Design review of the part built by this model. Coordinates are the model's own, in mm. Face numbers are marked on the shaded views. A direction names the side the tool comes from. Coordinates: 2 decimals unless noted, no trailing zeros. Loops run counter-clockwise (first coordinate to the right, second up) from the corner with the lowest first, then second, coordinate; pieces in that order, holes last. Notation, with made-up numbers: M -7.5,-26 L 3.5,-26 A14 cw 3.5,-5 Z; hole C 83,2 d3. An arc over 180 degrees is marked long. Put each result on its own line as item: value. Start each with the question number.
(1) Clearance check with flat-ended pins moving along their axes: pin 1 (2 mm diameter, centred on x = 2.5, z = 1.5, fed in from -Y); pin 2 (3.5 mm diameter, centred on x = -3.94, y = 8.65, fed in from +Z); pin 3 (0.9 mm diameter, centred on x = 1, z = 1, fed in from +Y); pin 4 (3 mm diameter, centred on y = 11.5, z = 1, fed in from +X). State where each tip first meets the part, or that it passes through.
(2) For the marked faces 5, 6, 7 and 8, list the 3-axis set-ups (+Z, -Z, +X, -X, +Y, -Y) from which the entire face can be reached by the end or side of a thin tool; tool diameter is ignored.
(3) Take a section at C-C, the plane y = 7.5. Give the boundary of the cut face in (x, z).
(4) Take a section at A-A, the plane x = -3.5. Give the boundary of the cut face in (y, z), then the cut area to 3 significant figures.
(5) The part is to be moulded in two halves that separate along Y. For the marked faces 1, 2, 3 and 4, say which applies: +Y half, -Y half, draft (parallel to the pull), parting line (faces both ways), or undercut.
(6) Take a section at D-D, the plane z = 1. Give the boundary of the cut face in (x, y), then the cut area to 3 significant figures.
(7) For probe 1 along X at (y, z) = (9.5, 0.25); probe 2 along X at (y, z) = (8, -1); probe 3 along Y at (x, z) = (-3.75, -3), list the stretches that pass through material, from the lowest coordinate up. Write a range as [from, to].
(8) Take a section at B-B, the plane z = -0.75. Give the boundary of the cut face in (x, y).
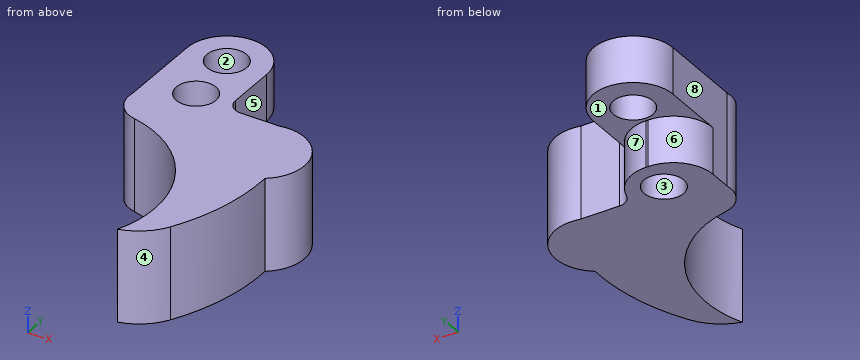
```python
from build123d import *

# Parameters (mm, degrees)
BOSS_EXTRUDE1_DEPTH      = 3.5
BOSS_EXTRUDE1_DEPTH_BACK = 3.5
SKETCH6_R                = 1.5
CUT_EXTRUDE1_DEPTH       = 19.96660999
SKETCH7_W                = 4.034122634
SKETCH7_H                = 6.882168449
CUT_EXTRUDE2_DEPTH       = 18.97170817
FILLET1_R                = 3
CUT_EXTRUDE3_DEPTH       = 18.97170817
CUT_EXTRUDE3_DEPTH_BACK  = 18.97170817
SKETCH5_R                = 1.5


with BuildPart() as part:
    # Sketch1 → Boss-Extrude1 (new, two sides: drawn at the far end of the back side and taken through both)
    with BuildSketch(Plane.XY.offset(-BOSS_EXTRUDE1_DEPTH_BACK)):
        with BuildLine():
            Line((-7.379331989, 6.554089817), (-7.379331989, 12.992324067))
            ThreePointArc((-7.379331989, 12.992324067), (-4.379331989, 15.992324067), (-1.379331989, 12.992324067))
            Line((-1.379331989, 12.992324067), (-1.379331989, 9.288226288))
            ThreePointArc((-1.379331989, 9.288226288), (-1.067058002, 8.534330194), (-0.313161909, 8.222056208))
            Line((-0.313161909, 8.222056208), (2.596292865, 8.222056208))
            ThreePointArc((2.596292865, 8.222056208), (6.230009224, 6.392230094), (5.19642183, 2.457277072))
            ThreePointArc((5.19642183, 2.457277072), (4.763363262, -1.740328915), (3.218784408, -5.667377669))
            ThreePointArc((3.218784408, -5.667377669), (2.087900651, -6.964096239), (0.531658525, -7.697913361))
            ThreePointArc((0.531658525, -7.697913361), (0.209560398, -0.37433078), (-5.652587934, 4.027240071))
            ThreePointArc((-5.652587934, 4.027240071), (-7.035324124, 4.93575307), (-7.379331989, 6.554089817))
        make_face()
    extrude(amount=BOSS_EXTRUDE1_DEPTH + BOSS_EXTRUDE1_DEPTH_BACK)

    # Sketch6 → Cut-Extrude1 (cut, through all)
    with BuildSketch(Plane.XY.offset(3.5)):
        with Locations((-4.379331989, 12.992324067)):
            Circle(SKETCH6_R)
    extrude(amount=-CUT_EXTRUDE1_DEPTH, mode=Mode.SUBTRACT)

    # Sketch7 → Cut-Extrude2 (cut, through all)
    with BuildSketch(Plane(origin=(0, 0, 0), x_dir=(0, 0, -1), z_dir=(1, 0, 0))):
        with Locations((2.017061317, 14.662562736)):
            Rectangle(SKETCH7_W, SKETCH7_H)
    extrude(amount=-CUT_EXTRUDE2_DEPTH, mode=Mode.SUBTRACT)

    # Fillet1
    # the kernel refuses this fillet: 3 mm, written as the material it takes off along each edge
    with BuildSketch(Plane(origin=(-7.379331989, 11.221478511, 0), x_dir=(0, -1, 0), z_dir=(0, 0, -1))) as fillet1_piece_1:
        with BuildLine():
            CenterArc((FILLET1_R, -FILLET1_R), FILLET1_R, 90, 90)
            Line((0, -FILLET1_R), (0, 0))
            Line((0, 0), (FILLET1_R, 0))
        make_face()
    extrude(amount=11, mode=Mode.SUBTRACT)
    with BuildSketch(Plane(origin=(-1.379331989, 11.221478511, -10.643941593), x_dir=(0.016872794888794368, -0.9998576442637425, 0), z_dir=(0, 0, 1))) as fillet1_piece_2:
        with BuildLine():
            CenterArc((2.951357628, -2.907788229), FILLET1_R, 104.242588424, 74.790625764)
            Line((-0.048215304, -2.857169845), (-0.348172598, -2.852108006))
            Line((-0.348172598, -2.852108006), (-0.299957293, 0.005061838))
            Line((-0.299957293, 0.005061838), (0.005061838, 0.299957293))
            ThreePointArc((0.005061838, 0.299957293), (1.938038852, 0.267337925), (2.13946551, 0.290778823))
            Line((2.13946551, 0.290778823), (2.213273884, 0))
        make_face()
    extrude(amount=10.643941593, mode=Mode.SUBTRACT)

    # Sketch5 → Cut-Extrude3 (cut, two sides: drawn at the far end of the back side and taken through both)
    with BuildSketch(Plane.XY.offset(-CUT_EXTRUDE3_DEPTH_BACK)):
        with Locations((-3.938565523, 8.651692055)):
            Circle(SKETCH5_R)
    extrude(amount=CUT_EXTRUDE3_DEPTH + CUT_EXTRUDE3_DEPTH_BACK, mode=Mode.SUBTRACT)


solid = part.part
```
Computed values:
1. pin 1: stops at y = -7.34
1. pin 2: stops at z = 3.5
1. pin 3: stops at y = 8.22
1. pin 4: stops at x = -1.38
2. face 5: +Z, -Z, +X, +Y
2. face 6: -Z, -X, +Y
2. face 7: -Z, +X, +Y
2. face 8: +Z, -Z, -X, +Y
3. outline: M -7.38,-3.5 L -4.9,-3.5 L -4.9,3.5 L -7.38,3.5 Z; M -2.98,-3.5 L 5.41,-3.5 L 5.41,3.5 L -2.98,3.5 Z
4. outline: M 3.28,-3.5 L 7.22,-3.5 L 7.22,3.5 L 3.28,3.5 Z; M 10.09,-3.5 L 11.13,-3.5 L 11.13,0 L 11.78,0 L 11.78,3.5 L 10.09,3.5 Z; M 14.21,0 L 15.86,0 L 15.86,3.5 L 14.21,3.5 Z
4. area: 42.9 mm^2
5. face 1: draft
5. face 2: undercut
5. face 3: undercut
5. face 4: -Y half
6. outline: M -7.38,6.55 A2.18 ccw -5.65,4.03 A8.58 cw 0.53,-7.7 A4.2 ccw 3.22,-5.67 A15.57 ccw 5.2,2.46 A3.23 ccw 2.6,8.22 L -0.31,8.22 A1.07 cw -1.38,9.29 L -1.38,12.99 A3 ccw -7.38,12.99 Z; hole C -4.38,12.99 d3; hole C -3.94,8.65 d3
6. area: 137 mm^2
7. probe 1: x = [-7.38, -5.18], [-2.7, -1.38]
7. probe 2: x = [-7.38, -5.29], [-2.59, 4.63]
7. probe 3: y = [3.4, 7.16], [10.14, 11.18]
8. outline: M -7.38,6.55 A2.18 ccw -5.65,4.03 A8.58 cw 0.53,-7.7 A4.2 ccw 3.22,-5.67 A15.57 ccw 5.2,2.46 A3.23 ccw 2.6,8.22 L -0.31,8.22 A1.07 cw -1.34,9.01 A3 ccw -4.24,11.22 L -4.38,11.22 A3 ccw -7.38,8.22 Z; hole C -3.94,8.65 d3
